Part print with two shaded views. Sizes in mm from the minimum x, y, z corner. A direction names the side the tool comes from. Round coordinates to 2 decimals unless told otherwise and drop trailing zeros. Order: outer loops, then holes, each group sorted by start corner. A loop starts at its lowest first (then second) coordinate and runs counter-clockwise, first axis right, second up. Notation, with made-up numbers: (22.25, 28) -> (52.25, 28) arc R20 ccw to (52.25, 56) -> close; hole circle Ø4 at (27, -21.75). An arc over 180 degrees is marked (long way). Put each result on its own line as item: value. Start each with the question number.
Q1. Pull direction X, two halves, no side cores. Call the marked faces 4, 5, 6 and 7: released by +X, released by -X, zero draft, split by the parting line, or undercut.
Q2. Cut at D-D, the plane x = 28. List the corners of the cut face in (y, z) (1 decimal).
Q3. Flat gauge pins, fed straight in: P1, Ø3, axis at x = 45, y = 34.5, coming from the +Z side (1 decimal); P2, Ø1.5, axis at x = 18.5, z = 29, coming from the -Y side; P3, Ø5.5, axis at x = 31, z = 19, coming from the +Y side. Where does each tip first touch, or does it go through?
Q4. Cut at B-B, the plane z = 13. List the corners of the cut face in (x, y), and give its area (3 significant figures).
Q5. Probe L1, parallel to Z at x = 38, y = 16.5; L2, parallel to Y at x = 36.5, z = 29; L3, parallel to X at y = 100.5, z = 41 (1 decimal). List the from-to ranges inside material, lowest first.
Q6. Cut at C-C, the plane y = 124.5. List the corners of the cut face in (x, z) (1 decimal), and give its area (3 significant figures).
Q7. 3-axis set-ups, long thin cutter, end or side, ignore diameter. For the marked faces 1, 2 and 3: which of +Z, -Z, +X, -X, +Y, -Y reach the whole face in a straight line?
Q8. Cut at A-A, the plane x = 42. List the corners of the cut face in (y, z) (1 decimal), and give its area (3 significant figures).
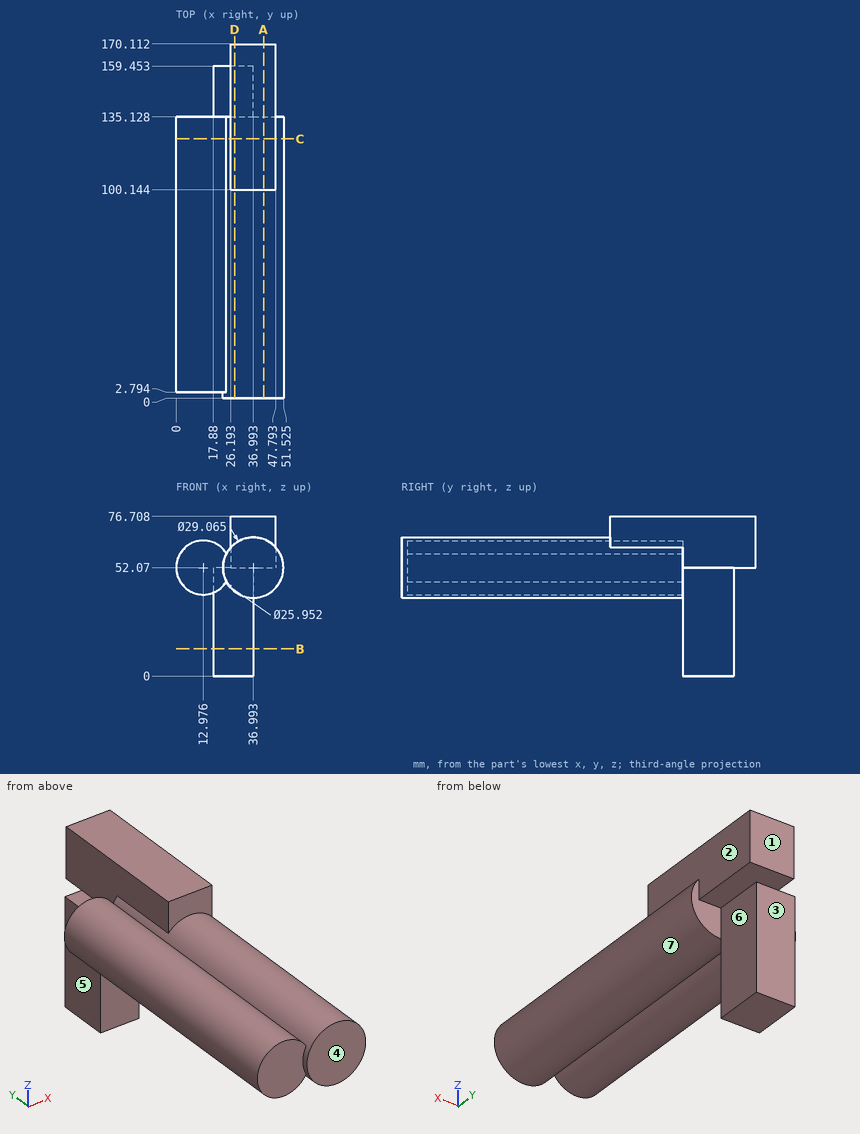
Ans:
1. face 4: zero draft
1. face 5: released by -X
1. face 6: released by +X
1. face 7: undercut
2. outline: (0, 40.7) -> (135.1, 40.7) -> (135.1, 0) -> (159.5, 0) -> (159.5, 52.1) -> (170.1, 52.1) -> (170.1, 76.7) -> (100.1, 76.7) -> (100.1, 63.5) -> (0, 63.5) -> close
3. P1: stops at z = 65.1
3. P2: stops at y = 135.13
3. P3: stops at y = 159.45
4. outline: (17.88, 135.13) -> (36.99, 135.13) -> (36.99, 159.45) -> (17.88, 159.45) -> close
4. area: 465 mm^2
5. L1: z = 37.57 to 66.57
5. L2: y = 135.13 to 159.45
5. L3: x = 6.2 to 19.7, 27.6 to 46.4
6. outline: (24.1, 45.4) arc R14.5 ccw (long way) to (47.8, 61.8) -> (47.8, 76.7) -> (26.2, 76.7) -> (26.2, 61.8) arc R14.5 ccw to (24.1, 58.8) arc R13 ccw (long way) to start
6. area: 1,410 mm^2
7. face 1: +Z, -Z, +X, -X, +Y
7. face 2: +Z, +X, +Y
7. face 3: -Z, +X, -X, +Y
8. outline: (0, 38.4) -> (135.1, 38.4) -> (135.1, 52.1) -> (170.1, 52.1) -> (170.1, 76.7) -> (100.1, 76.7) -> (100.1, 65.7) -> (0, 65.7) -> close
8. area: 4,930 mm^2
